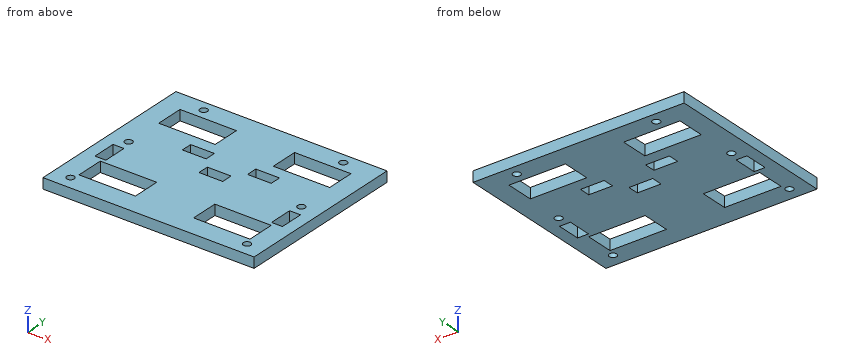
from build123d import *

# Parameters (mm, degrees)
SKETCH1_W           = 90.75
SKETCH1_H           = 75
SKETCH1_W_2         = 24.25
SKETCH1_H_2         = 12
BOSS_EXTRUDE1_DEPTH = 4.5
SKETCH2_R           = 1.6
SCREWHOLES_DEPTH    = 60.037196961
SKETCH3_W           = 10.2
SKETCH3_H           = 4.7
BELTCLAMP_DEPTH     = 60.037196961
SKETCH4_W           = 10.2
SKETCH4_H           = 4.7
CUT_EXTRUDE3_DEPTH  = 60.037196961
SKETCH5_R           = 1.6
SKETCH5_W           = 4.7
SKETCH5_H           = 10.2
CUT_EXTRUDE4_DEPTH  = 60.037196961


with BuildPart() as part:
    # Sketch1 → Boss-Extrude1 (new body)
    with BuildSketch(Plane.XY):
        Rectangle(SKETCH1_W, SKETCH1_H)
        with Locations((-24.625, 22.5)):
            Rectangle(SKETCH1_W_2, SKETCH1_H_2, mode=Mode.SUBTRACT)
        with Locations((24.625, 22.5)):
            Rectangle(SKETCH1_W_2, SKETCH1_H_2, mode=Mode.SUBTRACT)
        with Locations((24.625, -22.5)):
            Rectangle(SKETCH1_W_2, SKETCH1_H_2, mode=Mode.SUBTRACT)
        with Locations((-24.625, -22.5)):
            Rectangle(SKETCH1_W_2, SKETCH1_H_2, mode=Mode.SUBTRACT)
    extrude(amount=BOSS_EXTRUDE1_DEPTH)

    # Sketch2 → screwHoles (cut, through all)
    with BuildSketch(Plane.XY.offset(4.5)):
        with Locations((-30, 33)):
            Circle(SKETCH2_R)
        with Locations(Location((30, 33, 0), (0, 0, 180))):
            Circle(SKETCH2_R)
        with Locations((37.125, 0)):
            Circle(SKETCH2_R)
        with Locations(Location((-37.125, 0, 0), (0, 0, 180))):
            Circle(SKETCH2_R)
    extrude(amount=-SCREWHOLES_DEPTH, mode=Mode.SUBTRACT)

    # Sketch3 → BeltClamp (cut, through all)
    with BuildSketch(Plane.XY.offset(4.5)):
        with Locations((-14, 9)):
            Rectangle(SKETCH3_W, SKETCH3_H)
        with Locations((14, 9)):
            Rectangle(SKETCH3_W, SKETCH3_H)
    extrude(amount=-BELTCLAMP_DEPTH, mode=Mode.SUBTRACT)

    # Sketch4 → Cut-Extrude3 (cut, through all)
    with BuildSketch(Plane.XY.offset(4.5)):
        Rectangle(SKETCH4_W, SKETCH4_H)
    extrude(amount=-CUT_EXTRUDE3_DEPTH, mode=Mode.SUBTRACT)

    # Sketch5 → Cut-Extrude4 (cut, through all)
    with BuildSketch(Plane.XY.offset(4.5)):
        with Locations((37.95, -31.75)):
            Circle(SKETCH5_R)
        with Locations(Location((-37.95, -31.75, 0), (0, 0, 180))):
            Circle(SKETCH5_R)
        with Locations((37.95, -9.75)):
            Rectangle(SKETCH5_W, SKETCH5_H)
        with Locations((-37.95, -9.75)):
            Rectangle(SKETCH5_W, SKETCH5_H)
    extrude(amount=-CUT_EXTRUDE4_DEPTH, mode=Mode.SUBTRACT)


solid = part.part
Check sheet for the modelled part. Datum: model origin and axes. Units: mm. Round coordinates to 2 decimals unless told otherwise and drop trailing zeros. Order: outer loops, then holes, each group sorted by start corner. A loop starts at its lowest first (then second) coordinate and runs counter-clockwise, first axis right, second up.
Q1. Cross-section at A-A, the plane x = -26.5. Enter the section's corners in (y, z).
Filled sheet:
outline: (-37.5, 0) - (-28.5, 0) - (-28.5, 4.5) - (-37.5, 4.5) - close; (-16.5, 0) - (16.5, 0) - (16.5, 4.5) - (-16.5, 4.5) - close; (28.5, 0) - (37.5, 0) - (37.5, 4.5) - (28.5, 4.5) - close
Q2. Cross-section at D-D, the plane x = -3. Enter the section's corners in (y, z), plus the area to 3 significant figures.
Filled sheet:
outline: (-37.5, 0) - (-2.35, 0) - (-2.35, 4.5) - (-37.5, 4.5) - close; (2.35, 0) - (37.5, 0) - (37.5, 4.5) - (2.35, 4.5) - close
area: 316 mm2
Q3. Cross-section at C-C, the plane y = -31.75. Enter the section's corners in (x, z) (3 decimals).
Filled sheet:
outline: (-45.375, 0) - (-39.55, 0) - (-39.55, 4.5) - (-45.375, 4.5) - close; (-36.35, 0) - (36.35, 0) - (36.35, 4.5) - (-36.35, 4.5) - close; (39.55, 0) - (45.375, 0) - (45.375, 4.5) - (39.55, 4.5) - close
Q4. Cross-section at B-B, the plane x = 17.5. Enter the section's corners in (y, z), plus the area to 3 significant figures.
Filled sheet:
outline: (-37.5, 0) - (-28.5, 0) - (-28.5, 4.5) - (-37.5, 4.5) - close; (-16.5, 0) - (6.65, 0) - (6.65, 4.5) - (-16.5, 4.5) - close; (11.35, 0) - (16.5, 0) - (16.5, 4.5) - (11.35, 4.5) - close; (28.5, 0) - (37.5, 0) - (37.5, 4.5) - (28.5, 4.5) - close
area: 208 mm2
Q5. Scan lines: L1, parallel to Y at x = -16, z = 1.25; L2, parallel to X at y = -5, z = 2.35 (3 decimals); L3, parallel to Y at x = -27.5, z = 3.6. Record each from-to range of solid material in increasing order.
Filled sheet:
L1: y = -37.5 to -28.5, -16.5 to 6.65, 11.35 to 16.5, 28.5 to 37.5
L2: x = -45.375 to -40.3, -35.6 to 35.6, 40.3 to 45.375
L3: y = -37.5 to -28.5, -16.5 to 16.5, 28.5 to 37.5
Q6. Depth check by flat-ended pin: P1, Ø2.5, axis at x = -37.95, y = -31.75, coming from the -Z side. Enter the tip coordinate at first touch or a pass-through.
Filled sheet:
P1: passes through
